Geometry: final body of the model. Coordinates: model frame, mm. A direction names the side the tool comes from. Give positions to 0.01 mm unless a question says otherwise; leave off trailing zeros. Order: outer loops, then holes, each group sorted by start corner. A loop starts at its lowest first (then second) coordinate and runs counter-clockwise, first axis right, second up. Notation, with made-up numbers: (-22.75, -2.5) -> (4.25, -2.5) arc R12 ccw to (4.25, 11.5) -> close; hole circle Ø10 at (-27.5, 18.25). An arc over 180 degrees is marked (long way). One line per question, with ' | ' between items. Start each with the question number.
(1) Section B-B (z = 61.5). Return loops of the section in (x, y), then the cut area to 3 significant figures.
(2) Set-up query: faces 1 (the face through (-38, -3, 25.098)), 2 (the face through (-67.27, -2.5, 55.35)), 3 (the face through (0, 0, 0)), 4 (the face through (-76.143, -3, 72)). Return all of +Z, -Z, +X, -X, +Y, -Y with unobstructed straight access to the full face (end or side cutting, diameter ignored); none if empty.
(3) Ray query, L1, parallel to X at y = 14, z = 10; L2, parallel to X at y = -6, z = 55.5; L3, parallel to Y at x = -1.5, z = 77. Return the intervals inside material, ascending.
(4) First-contact query: pin 1 Ø3 at (x, z) = (-22, 20) entering from -Y; pin 2 Ø1.5 at (x, y) = (-10.5, -1) entering from +Z; pin 3 Ø3 at (y, z) = (-25.5, 41.5) entering from -X. Flat tips, straight axial feed; report the tip coordinate or a pass-through.
(5) Mould query, pull axis X, two halves, no side actions, for faces 5 (the face through (-71, -5.08, 56)), 6 (the face through (-69.593, -2.504, 84.412)), 7 (the face through (-47.347, -2.504, 82.146)). Classes: +X half, -X half, draft (parallel to the pull), parting line (faces both ways), or undercut.
(6) Section C-C (z = 23). Return loops of the section in (x, y).
(7) Section A-A (z = 13.5). Return loops of the section in (x, y), then the cut area to 3 significant figures.
```python
from build123d import *

# Parameters (mm, degrees)
F3_DEPTH = 5.08
F4_R     = 2.54


with BuildPart() as f1:
    # F0 (on Front) → F1 (revolve)
    with BuildSketch(Plane.XZ):
        Polygon((-32, 0), (0, 0), (0, 5), (-27.64709, 5), (-40.047639, 94.188564), (-45, 93.5), align=None)
        Polygon((-27.64709, 5), (0, 5), (-16.727764, 16.835798), align=None)
    revolve(axis=Axis((0, 0, 46.75), (0, 0, 1)))

    # F2 (on Front) → F3 (join)
    with BuildSketch(Plane.XZ):
        with BuildLine():
            ThreePointArc((-68.295348, 59.845981), (-66.09924, 72.713495), (-53.492135, 76.098273))
            ThreePointArc((-53.492135, 76.098273), (-51.366423, 75.191833), (-49.451803, 73.897802))
            Line((-49.451803, 73.897802), (-41.887928, 69.778316))
            Line((-41.887928, 69.778316), (-42.81877, 80.389924))
            Line((-42.81877, 80.389924), (-51.94103, 83.927125))
            Line((-51.94103, 83.927125), (-59.015434, 85.788816))
            Line((-59.015434, 85.788816), (-67.206852, 85.788816))
            Line((-67.206852, 85.788816), (-72.047234, 82.996286))
            Line((-72.047234, 82.996286), (-76.142944, 77.597402))
            Line((-76.142944, 77.597402), (-76.142944, 72.943188))
            Line((-76.142944, 72.943188), (-76.142944, 66.985793))
            Line((-76.142944, 66.985793), (-77.259958, 63.07625))
            Line((-77.259958, 63.07625), (-76.329112, 57.491191))
            Line((-76.329112, 57.491191), (-76.329112, 53.209316))
            Line((-76.329112, 53.209316), (-73.72275, 50.230619))
            Line((-73.72275, 50.230619), (-71.488731, 46.507247))
            Line((-71.488731, 46.507247), (-66.462182, 38.874336))
            Line((-66.462182, 38.874336), (-62.366471, 33.475447))
            Line((-62.366471, 33.475447), (-57.712257, 31.61376))
            Line((-57.712257, 31.61376), (-51.568694, 28.821234))
            Line((-51.568694, 28.821234), (-45.797467, 27.145715))
            Line((-45.797467, 27.145715), (-39.467737, 25.097862))
            Line((-39.467737, 25.097862), (-35.558198, 25.097862))
            Line((-35.558198, 25.097862), (-37.047546, 34.406289))
            Line((-37.047546, 34.406289), (-43.563444, 36.267977))
            Line((-43.563444, 36.267977), (-51.754862, 40.363684))
            Line((-51.754862, 40.363684), (-59.760112, 42.783875))
            Line((-59.760112, 42.783875), (-66.276014, 50.975293))
            Line((-66.276014, 50.975293), (-68.295348, 59.845981))
        make_face()
        with BuildLine():
            ThreePointArc((-49.451803, 73.897802), (-51.366423, 75.191833), (-53.492135, 76.098273))
            Line((-53.492135, 76.098273), (-49.451803, 73.897802))
        make_face()
    extrude(amount=F3_DEPTH)

    # F4
    f4_edges = [f1.edges().sort_by_distance(p)[0] for p in [
        (40.047639, 0, 94.188564),
    ]]
    fillet(f4_edges, radius=F4_R)


solid = f1.part
```
Response:
1) outline: (-77, -5.08) -> (-68.86, -5.08) -> (-68.86, 0) -> (-77, 0) -> close; circle Ø81.1 at (0, 0); hole circle Ø71.01 at (0, 0) | area: 1,250 mm^2
2) face 1: -Z, -X, +Y, -Y | face 2: +Y, -Y | face 3: -Z, +X, -X, +Y, -Y | face 4: +Z, -X, +Y, -Y
3) L1: x = -30.31 to -24.64, -18.29 to 18.29, 24.64 to 30.31 | L2: x = -39.26 to -34.15, 34.15 to 39.26 | L3: y = -42.68 to -37.63, 37.63 to 42.68
4) pin 1: stops at y = -28.13 | pin 2: stops at z = 12.99 | pin 3: stops at x = -29.19
5) face 5: draft | face 6: -X half | face 7: undercut
6) outline: circle Ø70.4 at (0, 0); hole circle Ø60.3 at (0, 0)
7) outline: circle Ø67.75 at (0, 0); circle Ø39.61 at (0, 0); hole circle Ø57.66 at (0, 0); hole circle Ø24.03 at (0, 0) | area: 1,770 mm^2
